Can you work these out from the model? Positions are in its coordinate system, mm. A direction names the side the tool comes from. Give positions to 0.01 mm unless a question says otherwise; leave off trailing zeros. Loops run counter-clockwise (first coordinate to the right, second up) from the corner with the lowest first, then second, coordinate; pieces in that order, holes last. Notation, with made-up numbers: (-8.5, 26) -> (7.5, 26) arc R14 cw to (7.5, 40) -> close; hole circle Ø10 at (85.25, 46.25). An arc over 180 degrees is marked (long way). Return JSON: item names as keys, results as strings. Group by question number.
Q1. Suppose I cut it at D-D, the plane y = -22. Please give me the cut outline in (x, z), and give its area (3 significant figures).
Q2. Thinking about a two-plate mould opening in Y: for faces 1 (the flat face through (-1, 42.925, 6)), 2 (the flat face through (-16, 20, 13)), 3 (the flat face through (-14, -32.8, 7)), which applies, pulls with the +Y half, pulls with the -Y half, needs draft (parallel to the pull), parting line crosses it, or undercut?
Q3. Will these pins go through, and if not, where does the flat tip stop? pin 1 (3 mm diameter, centred on x = -10, y = -14, fed in from +Z); pin 2 (10 mm diameter, centred on x = -22.5, y = 8.5, fed in from -Z); pin 3 (3.5 mm diameter, centred on y = 34.925, z = 6.5, fed in from -X).
Q4. Suppose I cut it at B-B, the plane z = 6.5. Count the separate pieces of the cut face and the enclosed holes in it, and give its area (3 significant figures).
Q5. Which directions (+Z, -Z, +X, -X, +Y, -Y) give clear straight access to the entire face, cutting with the end or side of a thin tool? Please do faces 4 (the flat face through (66.45, -1, 6)), 5 (the flat face through (-14, 32.8, 7)), 6 (the cylindrical face through (-54.12, -31.95, 6.11)).
Q6. I need wall thicknesses on line 1 along Y through (x, z) = (-33.95, 10.25) (3 decimals); line 2 along Y through (x, z) = (-49.5, 6.5) (3 decimals); line 3 along X through (y, z) = (7, 4). Which ranges of each line are inside material? Lowest first, please. Write a range as [from, to].
Q7. Suppose I cut it at A-A, the plane x = -27. Please give me the cut outline in (y, z) (3 decimals), and give its area (3 significant figures).
Q8. Suppose I cut it at C-C, the plane x = 39. Please give me the cut outline in (y, z) (3 decimals), and give its area (3 significant figures).
```python
from build123d import *

# Parameters (mm, degrees)
SZKIC1_W                    = 132.9
SZKIC1_H                    = 85.85
DODANIE_WYCI_GNI_CIE1_DEPTH = 13
SZKIC2_R                    = 36.5
SZKIC2_W                    = 5
SZKIC2_H                    = 73
WYTNIJ_WYCI_GNI_CIE1_DEPTH  = 2
WYTNIJ_WYCI_GNI_CIE3_DEPTH  = 13
SZYK_LINIOWY1_COUNT         = 2
SZYK_LINIOWY1_PITCH         = 69.6
SZYK_LINIOWY1_COUNT_DIR2    = 2
SZYK_LINIOWY1_PITCH_DIR2    = 69.6
WYTNIJ_WYCI_GNI_CIE4_DEPTH  = 13
SZKIC7_R                    = 11
WYTNIJ_WYCI_GNI_CIE5_DEPTH  = 13
SZKIC8_R                    = 3
WYTNIJ_WYCI_GNI_CIE6_DEPTH  = 25


with BuildPart() as part:
    # Szkic1 → Dodanie-wyciągnięcie1 (new body)
    with BuildSketch(Plane.XY):
        Rectangle(SZKIC1_W, SZKIC1_H)
    extrude(amount=DODANIE_WYCI_GNI_CIE1_DEPTH)

    # Szkic2 → Wytnij-wyciągnięcie1 (cut)
    with BuildSketch(Plane.XY.offset(13)):
        with Locations((23.52, 0)):
            Circle(SZKIC2_R)
        with Locations((18.52, 0)):
            Circle(SZKIC2_R)
        with Locations((21.02, 0)):
            Rectangle(SZKIC2_W, SZKIC2_H)
    extrude(amount=-WYTNIJ_WYCI_GNI_CIE1_DEPTH, mode=Mode.SUBTRACT)

    # Szkic3 → Wytnij-wyciągnięcie3 (cut)
    with BuildSketch(Plane.XY.offset(13)):
        with BuildLine():
            ThreePointArc((55.325, 34.8), (54.739213562, 36.214213562), (53.325, 36.8))
            Line((53.325, 36.8), (53.325, 32.8))
            ThreePointArc((53.325, 32.8), (54.739213562, 33.385786438), (55.325, 34.8))
        make_face()
        with BuildLine():
            Line((53.325, 32.8), (53.325, 36.8))
            ThreePointArc((53.325, 36.8), (51.325, 34.8), (53.325, 32.8))
        make_face()
        with BuildLine():
            Line((58.325, 36.8), (53.325, 36.8))
            ThreePointArc((53.325, 36.8), (54.739213562, 36.214213562), (55.325, 34.8))
            ThreePointArc((55.325, 34.8), (54.739213562, 33.385786438), (53.325, 32.8))
            Line((53.325, 32.8), (58.325, 32.8))
            ThreePointArc((58.325, 32.8), (56.325, 34.8), (58.325, 36.8))
        make_face()
        with BuildLine():
            ThreePointArc((60.325, 34.8), (59.739213562, 36.214213562), (58.325, 36.8))
            Line((58.325, 36.8), (58.325, 32.8))
            ThreePointArc((58.325, 32.8), (59.739213562, 33.385786438), (60.325, 34.8))
        make_face()
        with BuildLine():
            Line((58.325, 32.8), (58.325, 36.8))
            ThreePointArc((58.325, 36.8), (56.325, 34.8), (58.325, 32.8))
        make_face()
    wytnij_wyci_gni_cie3 = extrude(amount=-WYTNIJ_WYCI_GNI_CIE3_DEPTH, mode=Mode.SUBTRACT)

    # Szyk liniowy1: Wytnij-wyci_gni_cie3 2 × 2
    with Locations(*[(-j * SZYK_LINIOWY1_PITCH_DIR2, -i * SZYK_LINIOWY1_PITCH, 0) for i in range(SZYK_LINIOWY1_COUNT) for j in range(SZYK_LINIOWY1_COUNT_DIR2) if (i, j) != (0, 0)]):
        add(wytnij_wyci_gni_cie3, mode=Mode.SUBTRACT)

    # Szkic6 → Wytnij-wyciągnięcie4 (cut)
    with BuildSketch(Plane.XY.offset(13)):
        with BuildLine():
            ThreePointArc((21.02, 8.645808233), (19.782482852, 8.911012123), (18.52, 9))
            Line((18.52, 9), (18.52, 7.483314774))
            ThreePointArc((18.52, 7.483314774), (19.725220987, 8.160860999), (21.02, 8.645808233))
        make_face()
        with BuildLine():
            Line((18.52, 7.483314774), (18.52, 9))
            ThreePointArc((18.52, 9), (9.52, 0), (18.52, -9))
            Line((18.52, -9), (18.52, -7.483314774))
            ThreePointArc((18.52, -7.483314774), (14.52, 0), (18.52, 7.483314774))
        make_face()
        with BuildLine():
            Line((18.52, -7.483314774), (18.52, -9))
            ThreePointArc((18.52, -9), (19.782482852, -8.911012123), (21.02, -8.645808233))
            ThreePointArc((21.02, -8.645808233), (19.725220987, -8.160860999), (18.52, -7.483314774))
        make_face()
        with BuildLine():
            Line((18.52, -7.483314774), (18.52, 7.483314774))
            ThreePointArc((18.52, 7.483314774), (14.52, 0), (18.52, -7.483314774))
        make_face()
        with BuildLine():
            ThreePointArc((21.02, 8.645808233), (19.725220987, 8.160860999), (18.52, 7.483314774))
            Line((18.52, 7.483314774), (18.52, -7.483314774))
            ThreePointArc((18.52, -7.483314774), (19.725220987, -8.160860999), (21.02, -8.645808233))
            ThreePointArc((21.02, -8.645808233), (22.314779013, -8.160860999), (23.52, -7.483314774))
            Line((23.52, -7.483314774), (23.52, 7.483314774))
            ThreePointArc((23.52, 7.483314774), (22.314779013, 8.160860999), (21.02, 8.645808233))
        make_face()
        with BuildLine():
            ThreePointArc((27.52, 0), (26.457253933, 4.242640687), (23.52, 7.483314774))
            Line((23.52, 7.483314774), (23.52, -7.483314774))
            ThreePointArc((23.52, -7.483314774), (26.457253933, -4.242640687), (27.52, 0))
        make_face()
        with BuildLine():
            ThreePointArc((32.52, 0), (29.883961031, 6.363961031), (23.52, 9))
            Line((23.52, 9), (23.52, 7.483314774))
            ThreePointArc((23.52, 7.483314774), (26.457253933, 4.242640687), (27.52, 0))
            ThreePointArc((27.52, 0), (26.457253933, -4.242640687), (23.52, -7.483314774))
            Line((23.52, -7.483314774), (23.52, -9))
            ThreePointArc((23.52, -9), (29.883961031, -6.363961031), (32.52, 0))
        make_face()
        with BuildLine():
            Line((23.52, 7.483314774), (23.52, 9))
            ThreePointArc((23.52, 9), (22.257517148, 8.911012123), (21.02, 8.645808233))
            ThreePointArc((21.02, 8.645808233), (22.314779013, 8.160860999), (23.52, 7.483314774))
        make_face()
        with BuildLine():
            ThreePointArc((21.02, -8.645808233), (22.257517148, -8.911012123), (23.52, -9))
            Line((23.52, -9), (23.52, -7.483314774))
            ThreePointArc((23.52, -7.483314774), (22.314779013, -8.160860999), (21.02, -8.645808233))
        make_face()
        with BuildLine():
            ThreePointArc((21.02, -8.645808233), (19.782482852, -8.911012123), (18.52, -9))
            Line((18.52, -9), (23.52, -9))
            ThreePointArc((23.52, -9), (22.257517148, -8.911012123), (21.02, -8.645808233))
        make_face()
        with BuildLine():
            Line((23.52, 9), (18.52, 9))
            ThreePointArc((18.52, 9), (19.782482852, 8.911012123), (21.02, 8.645808233))
            ThreePointArc((21.02, 8.645808233), (22.257517148, 8.911012123), (23.52, 9))
        make_face()
    extrude(amount=-WYTNIJ_WYCI_GNI_CIE4_DEPTH, mode=Mode.SUBTRACT)

    # Szkic7 → Wytnij-wyciągnięcie5 (cut)
    with BuildSketch(Plane.XY.offset(13)):
        with Locations((-33.95, 0)):
            Circle(SZKIC7_R)
    extrude(amount=-WYTNIJ_WYCI_GNI_CIE5_DEPTH, mode=Mode.SUBTRACT)

    # Szkic8 → Wytnij-wyciągnięcie6 (cut)
    with BuildSketch(Plane.ZY.offset(66.45)):
        with Locations((6.5, 34.925)):
            Circle(SZKIC8_R)
        with Locations((6.5, -34.925)):
            Circle(SZKIC8_R)
    extrude(amount=-WYTNIJ_WYCI_GNI_CIE6_DEPTH, mode=Mode.SUBTRACT)


solid = part.part
```
Ans:
{
 "1": {"outline": "(-66.45, 0) -> (66.45, 0) -> (66.45, 13) -> (52.64, 13) -> (52.64, 11) -> (-10.6, 11) -> (-10.6, 13) -> (-66.45, 13) -> close", "area": "1,600 mm^2"},
 "2": {"face 1": "pulls with the +Y half", "face 2": "needs draft", "face 3": "undercut"},
 "3": {"pin 1": "stops at z = 11", "pin 2": "stops at z = 0", "pin 3": "stops at x = -41.45"},
 "4": {"separate pieces": "1", "enclosed holes": "6", "area": "10,300 mm^2"},
 "5": {"face 4": "+Z, -Z, +X, +Y, -Y", "face 5": "+Z, -Z", "face 6": "-X"},
 "6": {"line 1": "y = [-42.925, -11], [11, 42.925]", "line 2": "y = [-42.925, -37.925], [-31.925, 31.925], [37.925, 42.925]", "line 3": "x = [-66.45, -42.44], [-25.46, 12.86], [29.18, 66.45]"},
 "7": {"outline": "(-42.925, 0) -> (-8.526, 0) -> (-8.526, 13) -> (-42.925, 13) -> close; (8.526, 0) -> (42.925, 0) -> (42.925, 13) -> (8.526, 13) -> close", "area": "894 mm^2"},
 "8": {"outline": "(-42.925, 0) -> (42.925, 0) -> (42.925, 13) -> (33.055, 13) -> (33.055, 11) -> (-33.055, 11) -> (-33.055, 13) -> (-42.925, 13) -> close", "area": "984 mm^2"}
}
